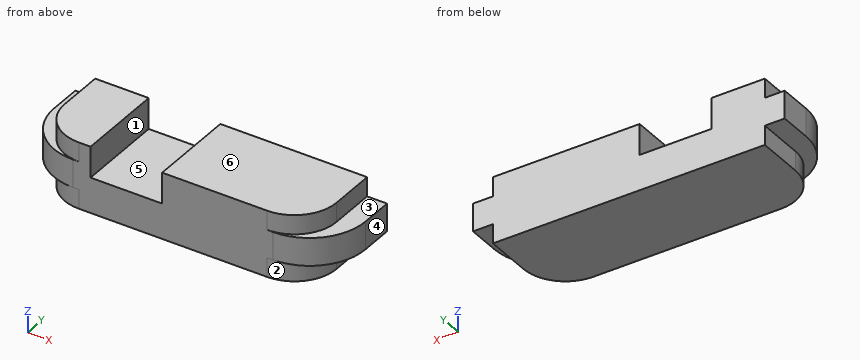
Solid Edge part; units mm, degrees
sketch "Sketch1" plane through (0, 0, 0) normal (0, -1, 0) x (1, 0, 0)
  line L0 (61.5, 15) -> (0, 15)
  line L1 (0, 15) -> (0, 10.65)
  line L2 (0, 10.65) -> (-4.5, 10.65)
  line L3 (-4.5, 10.65) -> (-4.5, 4.35)
  line L4 (0, 4.35) -> (-4.5, 4.35)
  line L5 (0, 0) -> (0, 4.35)
  line L6 (0, 0) -> (61.5, 0)
  line L7 (61.5, 0) -> (61.5, 4.35)
  line L8 (61.5, 4.35) -> (66, 4.35)
  line L9 (66, 10.65) -> (66, 4.35)
  line L10 (61.5, 10.65) -> (66, 10.65)
  line L11 (61.5, 15) -> (61.5, 10.65)
extrude "Protrusion1" add sketch "Sketch1" along normal blind 20
fillet "Round_2" radius 9.5 4 edges at (0, -20, 12.825) (0, -20, 2.175) (61.5, -20, 2.175) (61.5, -20, 12.825)
fillet "Round1" radius 12.65 2 edges at (-4.5, -20, 7.5) (66, -20, 7.5)
sketch "Sketch2" plane through (30.75, 0, 7.5) normal (0, 1, 0) x (1, 0, 0)
  line L0 (-2.44, -0.5) -> (-2.44, -7.5)
  line L1 (-2.59, -7.5) -> (-2.44, -7.5)
  line L2 (-18.49, -7.5) -> (-2.59, -7.5)
  line L3 (-18.64, -7.5) -> (-18.49, -7.5)
  line L4 (-18.64, -7.5) -> (-18.64, -0.5)
  line L5 (-18.64, -0.5) -> (-2.44, -0.5)
extrude "ExtrudedCutout_1" cut sketch "Sketch2" along normal mid plane 42.3972
Part model, mm, in its own coordinate system. Face numbers are marked on the shaded views. A direction names the side the tool comes from. Round coordinates to 2 decimals unless told otherwise and drop trailing zeros. Write each loop counter-clockwise with the first axis right and the second up, starting at its lowest first coordinate (ties: lowest second). Pieces come first, ordered by that corner, then holes. Notation, with made-up numbers: M -18.75,-37 L 7.25,-37 A4 ccw 7.25,-30 Z; hole C 55,61.5 d6. An arc over 180 degrees is marked long. Return JSON: item names as keys, results as strings. Group by question number.
(1) Saw through at A-A on z = 11.5. Write the cut outline in (x, y).
(2) Saw through at B-B on y = -6.5. Write the cut outline in (x, z), then the cut area to 3 significant figures.
(3) Saw through at C-C on x = 58.5. Write the cut outline in (y, z), then the cut area to 3 significant figures.
(4) Drill centre lines: probe 1 along X at (y, z) = (-3.25, 1); probe 2 along Z at (x, y) = (20, -7); probe 3 along X at (y, z) = (-7, 11.25). Where is each one in solid material? Low to high.
(5) Two-plate mould, pull along X, no slides. Class the marked faces 4, 5 and 6: +X half, -X half, draft (parallel to the pull), parting line (faces both ways), or undercut.
(6) Which spindle directions (+Z, -Z, +X, -X, +Y, -Y) get a long thin tool onto all of the face, cutting with end or side? Do the marked faces 1, 2 and 3. Say none if no direction does.
(7) Pin check, flat tips, straight feed: pin 1 Ø2 at (y, z) = (-12, 10) entering from -X; pin 2 Ø3.5 at (y, z) = (-2.5, 2.5) entering from +X; pin 3 Ø1.3 at (y, z) = (-5, 2) entering from -X. Stop position of each tip, or through.
(8) Saw through at D-D on z = 7. Write the cut outline in (x, y), then the cut area to 3 significant figures.
Returned:
{
 "1": {"outline": "M 0,-10.5 A9.5 ccw 9.5,-20 L 12.11,-20 L 12.11,0 L 0,0 Z; M 28.31,-20 L 52,-20 A9.5 ccw 61.5,-10.5 L 61.5,0 L 28.31,0 Z"},
 "2": {"outline": "M -4.5,4.35 L 0,4.35 L 0,0 L 61.5,0 L 61.5,4.35 L 66,4.35 L 66,10.65 L 61.5,10.65 L 61.5,15 L 28.31,15 L 28.31,8 L 12.11,8 L 12.11,15 L 0,15 L 0,10.65 L -4.5,10.65 Z", "area": "866 mm²"},
 "3": {"outline": "M -18.9,4.35 L -17.43,4.35 L -17.43,0 L 0,0 L 0,15 L -17.43,15 L -17.43,10.65 L -18.9,10.65 Z", "area": "271 mm²"},
 "4": {"probe 1": "0 to 61.5", "probe 2": "0 to 8", "probe 3": "0 to 12.11, 28.31 to 61.5"},
 "5": {"face 4": "+X half", "face 5": "undercut", "face 6": "draft"},
 "6": {"face 1": "+Z, +Y, -Y", "face 2": "-Z, +X, -Y", "face 3": "+Z, +X, -Y"},
 "7": {"pin 1": "x = -3.96", "pin 2": "x = 61.5", "pin 3": "x = 0"},
 "8": {"outline": "M -4.5,-7.35 A12.65 ccw 8.15,-20 L 53.35,-20 A12.65 ccw 66,-7.35 L 66,0 L -4.5,0 Z", "area": "1,340 mm²"}
}
